```python
from build123d import *

# Parameters (mm, degrees)
SKETCH1_W           = 650
SKETCH1_H           = 774.95
BOSS_EXTRUDE1_DEPTH = 10
SKETCH2_R           = 3
BOSS_EXTRUDE2_DEPTH = 10


with BuildPart() as part:
    # Sketch1 → Boss-Extrude1 (new body)
    with BuildSketch(Plane(origin=(0, 0, 0), x_dir=(1, 0, 0), z_dir=(0, 1, 0))):
        Rectangle(SKETCH1_W, SKETCH1_H)
    extrude(amount=BOSS_EXTRUDE1_DEPTH)

    # Sketch2 → Boss-Extrude2 (add)
    with BuildSketch(Plane.XZ):
        with Locations(Location((-203.532027454, 369.975, 0), (0, 0, 270))):
            Circle(SKETCH2_R)
        with Locations(Location((196.467972546, 369.975, 0), (0, 0, 270))):
            Circle(SKETCH2_R)
    boss_extrude2 = extrude(amount=BOSS_EXTRUDE2_DEPTH)

    # Mirror1: Boss-Extrude2 across plane
    add(boss_extrude2.mirror(Plane.XY))


solid = part.part
```
Work out the finished part from the listing and answer in its coordinate system (mm). Give positions to 0.01 mm unless a question says otherwise; leave off trailing zeros. Loops run counter-clockwise (first coordinate to the right, second up) from the corner with the lowest first, then second, coordinate; pieces in that order, holes last. Notation, with made-up numbers: (-40, 42) -> (4, 42) arc R19 ccw to (4, 49) -> close; hole circle Ø4 at (15, 35). An arc over 180 degrees is marked (long way). One line per question, with ' | ' between items. Start each with the question number.
1) A straight line is drawn through the part: L1, parallel to Y at x = -190, z = 94. Find the intervals that lie inside material, in ascending order.
2) This flat-tipped pin is pushed along its axis until it touches: pin 1 (1 mm diameter, centred on x = -91.5, z = 290.5, fed in from -Y). Where does it stop, or does it pass through?
3) Section C-C, the plane x = -95.5 is taken. Determine the outline of the cut face in (y, z) (3 decimals), then the cut area to 3 significant figures.
4) Section B-B, the plane y = -3.25 is taken. Determine the outline of the cut face in (x, z) (3 decimals).
5) Section A-A, the plane z = -23 is taken. Determine the outline of the cut face in (x, y).
Resolved:
1) L1: 0 to 10
2) pin 1: y = 0
3) outline: (0, -387.475) -> (10, -387.475) -> (10, 387.475) -> (0, 387.475) -> close | area: 7,750 mm2
4) outline: circle Ø6 at (-203.532, -369.975); circle Ø6 at (-203.532, 369.975); circle Ø6 at (196.468, -369.975); circle Ø6 at (196.468, 369.975)
5) outline: (-325, 0) -> (325, 0) -> (325, 10) -> (-325, 10) -> close
